Print and shaded views of the part. All mm, measured from the part's lowest x, y and z. Round coordinates to 2 decimals unless told otherwise and drop trailing zeros. Loops run counter-clockwise (first coordinate to the right, second up) from the corner with the lowest first, then second, coordinate; pieces in that order, holes last. Notation, with made-up numbers: (77, 19) -> (82, 19) arc R33 cw to (82, 55) -> close; hole circle Ø10 at (67.25, -19). An arc over 180 degrees is marked (long way). Answer as CSV lines item,"result".
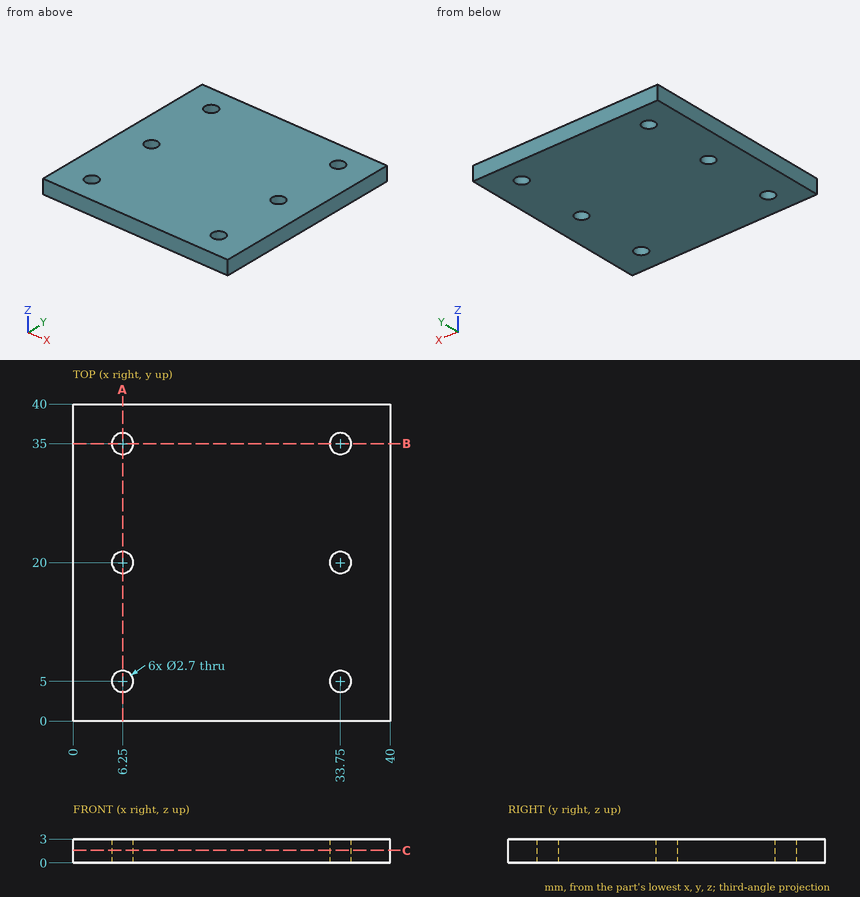
Q1. Slice it at B-B, the plane y = 35. Give the cut face in (x, z), and give its area (3 significant figures).
Results:
outline,"(0, 0) -> (4.9, 0) -> (4.9, 3) -> (0, 3) -> close; (7.6, 0) -> (32.4, 0) -> (32.4, 3) -> (7.6, 3) -> close; (35.1, 0) -> (40, 0) -> (40, 3) -> (35.1, 3) -> close"
area,"104 mm2"
Q2. Probe L1, parallel to Y at x = 6.25, z = 1.6; L2, parallel to X at y = 36, z = 1.8. List the from-to ranges inside material, lowest first. Write a range as [from, to].
Results:
L1,"[0, 3.65], [6.35, 18.65], [21.35, 33.65], [36.35, 40]"
L2,"[0, 5.34], [7.16, 32.84], [34.66, 40]"
Q3. Drop a flat-ended pin along its axis: pin 1 Ø3.5 at (x, y) = (33.75, 5) entering from +Z. Give the stop position or say it passes through.
Results:
pin 1,"z = 3"
Q4. Slice it at C-C, the plane z = 1.55. Give the cut face in (x, y), and give its area (3 significant figures).
Results:
outline,"(0, 0) -> (40, 0) -> (40, 40) -> (0, 40) -> close; hole circle Ø2.7 at (6.25, 5); hole circle Ø2.7 at (6.25, 20); hole circle Ø2.7 at (6.25, 35); hole circle Ø2.7 at (33.75, 5); hole circle Ø2.7 at (33.75, 20); hole circle Ø2.7 at (33.75, 35)"
area,"1,570 mm2"
Q5. Slice it at A-A, the plane x = 6.25. Give the cut face in (y, z).
Results:
outline,"(0, 0) -> (3.65, 0) -> (3.65, 3) -> (0, 3) -> close; (6.35, 0) -> (18.65, 0) -> (18.65, 3) -> (6.35, 3) -> close; (21.35, 0) -> (33.65, 0) -> (33.65, 3) -> (21.35, 3) -> close; (36.35, 0) -> (40, 0) -> (40, 3) -> (36.35, 3) -> close"
